Could you check a few things on this model? Use its own coordinates, in mm. A direction names the side the tool comes from. Round coordinates to 2 decimals unless told otherwise and drop trailing zeros. Write each loop counter-clockwise with the first axis right and the second up, starting at its lowest first coordinate (ties: lowest second). Pieces come first, ordered by that corner, then holes. Notation, with made-up numbers: (17, 64) -> (56, 64) arc R28 ccw to (56, 83) -> close; hole circle Ø8 at (-17.5, 37.25). An arc over 180 degrees is marked (long way). Return JSON: item names as keys, results as strings.
from build123d import *

# Parameters (mm, degrees)
F0_W     = 40
F0_H     = 50
F1_DEPTH = 4
F2_W     = 40
F2_H     = 50
F2_R     = 4.076244
F2_R_2   = 4.144667
F2_R_3   = 3.582064
F3_DEPTH = 4
F4_R     = 5
F5_R     = 5
F6_R     = 12.071068


with BuildPart() as f1:
    # F0 (on Front) → F1 (new body)
    with BuildSketch(Plane.XZ):
        with Locations((20, 25)):
            Rectangle(F0_W, F0_H)
    extrude(amount=F1_DEPTH)

    # F2 (on Top) → F3 (join)
    with BuildSketch(Plane.XY):
        with Locations((20, -25)):
            Rectangle(F2_W, F2_H)
        with Locations((9.746881, -25.751499)):
            Circle(F2_R, mode=Mode.SUBTRACT)
        with Locations((20.625249, -39.535552)):
            Circle(F2_R_2, mode=Mode.SUBTRACT)
        with Locations((29.604357, -15.743585)):
            Circle(F2_R_3, mode=Mode.SUBTRACT)
    extrude(amount=F3_DEPTH)

    # F4
    f4_edges = [f1.edges().sort_by_distance(p)[0] for p in [
        (20, -4, 4),
    ]]
    fillet(f4_edges, radius=F4_R)

    # F5
    f5_edges = [f1.edges().sort_by_distance(p)[0] for p in [
        (20, 0, 0),
    ]]
    fillet(f5_edges, radius=F5_R)

    # F6
    f6_edges = [f1.edges().sort_by_distance(p)[0] for p in [
        (0, -50, 2),
        (40, -50, 2),
        (40, -2, 50),
        (0, -2, 50),
    ]]
    fillet(f6_edges, radius=F6_R)


solid = f1.part
1) If I drill on probe 1 along Z at (x, y) = (10, -11); probe 2 along Y at (x, z) = (36, 45); probe 3 along Y at (x, z) = (18, 3), over which ranges is the centre line in solid material (lowest first)? Write a range as [from, to].
Return value:
{"probe 1": "[0, 4]", "probe 2": "[-4, 0]", "probe 3": "[-50, -42.74], [-36.33, -0.42]"}
2) I want a section at A-A, the plane x = 22.5. Please give me the cut outline in (y, z), and give its area (3 significant figures).
Return value:
{"outline": "(-50, 0) -> (-43.23, 0) -> (-43.23, 4) -> (-50, 4) -> close; (-35.84, 0) -> (-5, 0) arc R5 ccw to (0, 5) -> (0, 50) -> (-4, 50) -> (-4, 9) arc R5 cw to (-9, 4) -> (-35.84, 4) -> close", "area": "354 mm²"}
3) For faces 1 (the face through (20, -2, 1)), 2 (the face through (20, -4, 30)), which set-ups out of +Z, -Z, +X, -X, +Y, -Y let a thin tool reach every point of the face, with its end or its side?
Return value:
{"face 1": "-Z, +X, -X, +Y", "face 2": "+Z, +X, -X, -Y"}
4) Thinking about a two-plate mould opening in Y: for faces 3 (the face through (3.44, -46.37, 2.03)), 4 (the face through (33.02, -14.67, 1.97)), 5 (the face through (13.635, -24.527, 1.972)), 6 (the face through (0, -11, 3)), which applies, pulls with the +Y half, pulls with the -Y half, needs draft (parallel to the pull), parting line crosses it, or undercut?
Return value:
{"face 3": "pulls with the -Y half", "face 4": "undercut", "face 5": "undercut", "face 6": "needs draft"}
5) Will these pins go through, and if not, where does the flat tip stop? pin 1 Ø20 at (x, z) = (27, 25.5) entering from -Y; pin 2 Ø3 at (x, y) = (30.5, -31.5) entering from +Z; pin 3 Ø1 at (x, y) = (24, -6.5) entering from +Z.
Return value:
{"pin 1": "y = -4", "pin 2": "z = 4", "pin 3": "z = 5"}
6) I want a section at D-D, the plane z = 20. Please give me the cut outline in (x, y).
Return value:
{"outline": "(0, -4) -> (40, -4) -> (40, 0) -> (0, 0) -> close"}
7) I want a section at C-C, the plane x = 7.5. Please give me the cut outline in (y, z).
Return value:
{"outline": "(-49.1, 0) -> (-29.15, 0) -> (-29.15, 4) -> (-49.1, 4) -> close; (-22.35, 0) -> (-5, 0) arc R5 ccw to (0, 5) -> (0, 49.1) -> (-4, 49.1) -> (-4, 9) arc R5 cw to (-9, 4) -> (-22.35, 4) -> close"}
8) I want a section at B-B, the plane y = -25. Please give me the cut outline in (x, z).
Return value:
{"outline": "(0, 0) -> (5.74, 0) -> (5.74, 4) -> (0, 4) -> close; (13.75, 0) -> (40, 0) -> (40, 4) -> (13.75, 4) -> close"}
